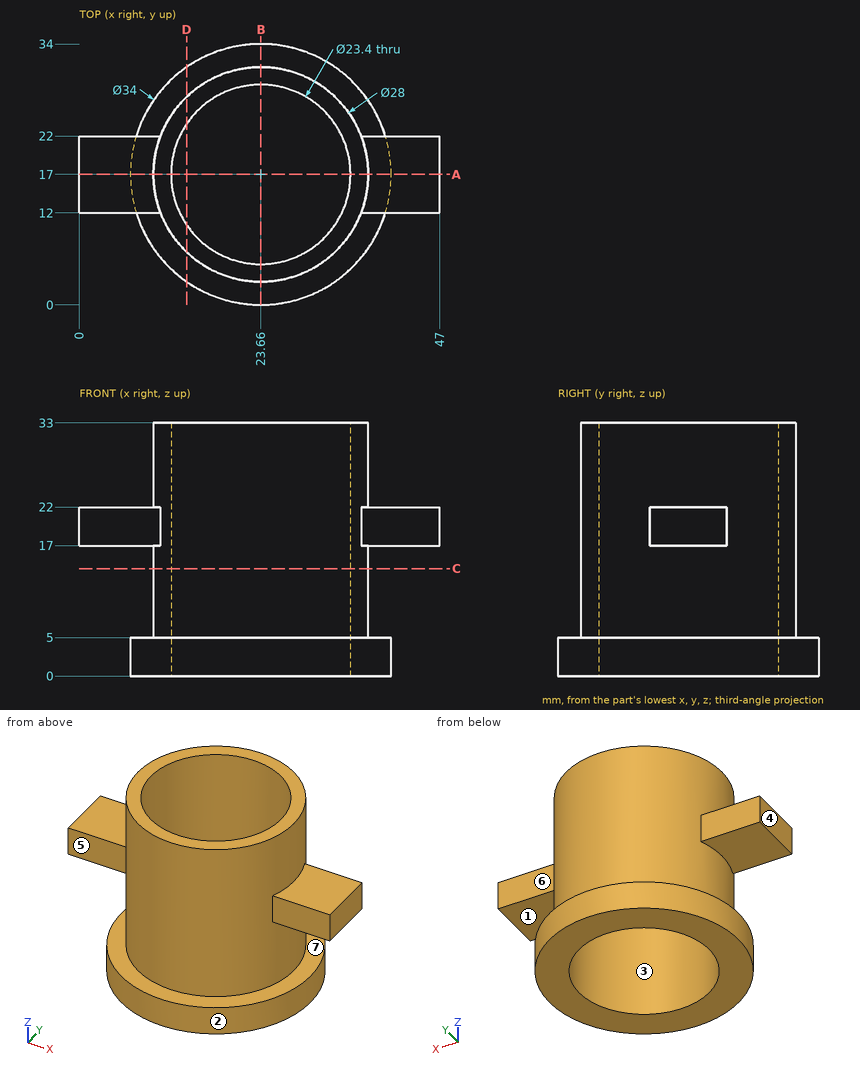
Here's the drawing with two shaded views (mm, measured from the low corner). I have some questions. A direction names the side the tool comes from. Round coordinates to 2 decimals unless told otherwise and drop trailing zeros. Loops run counter-clockwise (first coordinate to the right, second up) from the corner with the lowest first, then second, coordinate; pieces in that order, holes last.
1. Suppose I cut it at C-C, the plane z = 14. Please give me the cut outline in (x, y), and give its area (3 significant figures).
Answers:
outline: circle Ø28 at (23.66, 17); hole circle Ø23.4 at (23.66, 17)
area: 186 mm2
2. Thinking about a two-plate mould opening in X: for the marked faces 1, 2, 3 and 4, which applies, released by +X, released by -X, zero draft, split by the parting line, or undercut?
Answers:
face 1: zero draft
face 2: split by the parting line
face 3: undercut
face 4: released by -X
3. Suppose I cut it at B-B, the plane x = 23.66. Please give me the cut outline in (y, z).
Answers:
outline: (0, 0) - (5.3, 0) - (5.3, 33) - (3, 33) - (3, 5) - (0, 5) - close; (28.7, 0) - (34, 0) - (34, 5) - (31, 5) - (31, 33) - (28.7, 33) - close
4. Suppose I cut it at D-D, the plane x = 14. Please give me the cut outline in (y, z).
Answers:
outline: (3.01, 0) - (10.4, 0) - (10.4, 33) - (6.87, 33) - (6.87, 5) - (3.01, 5) - close; (23.6, 0) - (30.99, 0) - (30.99, 5) - (27.13, 5) - (27.13, 33) - (23.6, 33) - close
5. Will these pins go through, and if not, where does the flat tip stop? pin 1 (1.5 mm diameter, centred on y = 22.5, z = 19, fed in from -X); pin 2 (5.5 mm diameter, centred on x = 4.5, z = 18.5, fed in from +Y); pin 3 (8 mm diameter, centred on y = 30, z = 23, fed in from +X); pin 4 (3 mm diameter, centred on y = 12.5, z = 14.5, fed in from +X).
Answers:
pin 1: stops at x = 0
pin 2: stops at y = 22
pin 3: stops at x = 34.38
pin 4: stops at x = 37.33
6. If I drill on probe 1 along Y at (x, z) = (23.66, 20); probe 2 along X at (y, z) = (17.5, 16); probe 3 along Y at (x, z) = (32.5, 10.5), over which ranges is the centre line in solid material (lowest first)?
Answers:
probe 1: y = 3 to 5.3, 28.7 to 31
probe 2: x = 9.67 to 11.97, 35.35 to 37.65
probe 3: y = 6.14 to 9.34, 24.66 to 27.86
7. For the marked faces 5, 6 and 7, which set-ups out of +Z, -Z, +X, -X, +Y, -Y let a thin tool reach every point of the face, with its end or its side?
Answers:
face 5: +Z, -X, -Y
face 6: +Z, +X, +Y
face 7: none
8. Suppose I cut it at A-A, the plane y = 17. Please give me the cut outline in (x, z), and give its area (3 significant figures).
Answers:
outline: (0, 17) - (9.66, 17) - (9.66, 5) - (6.66, 5) - (6.66, 0) - (11.96, 0) - (11.96, 33) - (9.66, 33) - (9.66, 22) - (0, 22) - close; (35.36, 0) - (40.66, 0) - (40.66, 5) - (37.66, 5) - (37.66, 17) - (47, 17) - (47, 22) - (37.66, 22) - (37.66, 33) - (35.36, 33) - close
area: 277 mm2
